Autodesk Inventor part; units mm, degrees
ref_plane "YZ Plane" through (0, 0, 0) normal (1, 0, 0) x (0, 1, 0)
ref_plane "XZ Plane" through (0, 0, 0) normal (0, 1, 0) x (-1, 0, 0)
ref_plane "XY Plane" through (0, 0, 0) normal (0, 0, 1) x (1, 0, 0)
sketch "Эскиз1" plane through (0, 0, 0) normal (0, 0, 1) x (1, 0, 0)
  line L0 (-63, 0) -> (70, 0)
  line L1 (0, 29) -> (0, -30)
  circle A0 centre (35, 25) radius 1.25
  circle A1 centre (-22, 31) radius 1.25
  circle A2 centre (-22, -31) radius 1.25
  circle A3 centre (35, -25) radius 1.25
  arc A4 (31.0081, -7) -> (31.0081, 7) centre (46.5, 0) ccw
  line L2 (35, -25) -> (0, -25)
  circle A5 centre (25, -25) radius 1.5
  circle A6 centre (13, -25) radius 1.5
  arc A7 (31.0081, 7) -> (31.0081, -7) centre (35, 0) ccw
  line L3 (-44, 40) -> (74, 40)
  line L4 (80, 34) -> (80, -34)
  line L5 (-50, -34) -> (-50, 34)
  arc A8 (-44, 40) -> (-50, 34) centre (-44, 34) ccw
  arc A9 (-50, -34) -> (-44, -40) centre (-44, -34) ccw
  arc A10 (74, -40) -> (80, -34) centre (74, -34) ccw
  arc A11 (80, 34) -> (74, 40) centre (74, 34) ccw
  circle A12 centre (-44, 34) radius 2
  circle A13 centre (-44, -34) radius 2
  circle A14 centre (74, -34) radius 2
  circle A15 centre (74, 34) radius 2
  arc A16 (34.5621, -39.1892) -> (3.4379, -39.1892) centre (19, -66) ccw
  line L6 (74, -40) -> (37.5742, -40)
  line L7 (0.4258, -40) -> (-44, -40)
  arc A17 (0.4258, -40) -> (3.4379, -39.1892) centre (0.4258, -34) ccw
  arc A18 (34.5621, -39.1892) -> (37.5742, -40) centre (37.5742, -34) ccw
  point P0 (0, 0)
  point P1 (-50, 40)
  point P2 (80, 40)
  point P3 (80, -40)
  point P4 (-50, -40)
  point P5 (2.1181, -40)
  point P6 (35.8819, -40)
  dimension "d3" = 2.5
  dimension "d4" = 2.5
  dimension "d5" = 2.5
  dimension "d6" = 2.5
  dimension "d9" = 62
  dimension "d10" = 50
  dimension "d11" = 34
  dimension "d12" = 3
  dimension "d14" = 10
  dimension "d16" = 3
  dimension "d17" = 12
  dimension "d19" = 46.5
  dimension "d20" = 130
  dimension "d21" = 80
  dimension "d22" = 130
  dimension "d23" = 6
  dimension "d24" = 4
  dimension "d25" = 4
  dimension "d26" = 4
  dimension "d27" = 4
  dimension "d31" = 6
extrude "Выдавливание1" add sketch "Эскиз1" along normal blind 3
properties part number "06-01-Платформа для лидара"
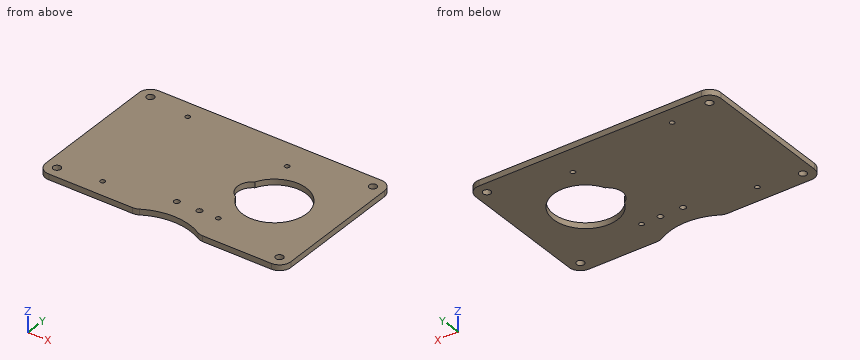
Could you check a few things on this model? Use its own coordinates, in mm. Coordinates: 2 decimals unless noted, no trailing zeros. Loops run counter-clockwise (first coordinate to the right, second up) from the corner with the lowest first, then second, coordinate; pieces in that order, holes last.
1. Imagine slicing it at C-C (y = -12). Please give me the cut outline in (x, z).
2. For P1, Ø2, axis at x = 35, y = 25, coming from the +Z side, with a flat end and sliding along its axis, tell me the tip position at first contact or that it passes through.
3. I need wall thicknesses on L1, parallel to X at y = -24, z = 2.2; L2, parallel to Y at x = 35, z = 0.6; L3, parallel to X at y = 15, z = 0.75. Which ranges of each line are inside material? Lowest first, please.
4. Imagine slicing it at B-B (x = 46.5). Please give me the cut outline in (y, z).
5. Imagine slicing it at A-A (z = 0.45). Give the number of separate pieces and of enclosed holes in the cut face, and give its area (3 significant figures).
Computed values:
1. outline: (-50, 0) - (34.46, 0) - (34.46, 3) - (-50, 3) - close; (58.54, 0) - (80, 0) - (80, 3) - (58.54, 3) - close
2. P1: passes through
3. L1: x = -50 to 11.88, 14.12 to 23.88, 26.12 to 34.25, 35.75 to 80
3. L2: y = -39.42 to -26.25, -23.75 to -12.52, 12.52 to 23.75, 26.25 to 40
3. L3: x = -50 to 38.5, 54.5 to 80
4. outline: (-40, 0) - (-17, 0) - (-17, 3) - (-40, 3) - close; (17, 0) - (40, 0) - (40, 3) - (17, 3) - close
5. separate pieces: 1
5. enclosed holes: 11
5. area: 9,240 mm2
